Read the model definition and answer for the solid it produces. Units are mm, in the model's axes. A direction names the side the tool comes from. Coordinates: 2 decimals unless noted, no trailing zeros. Loops run counter-clockwise (first coordinate to the right, second up) from the corner with the lowest first, then second, coordinate; pieces in that order, holes last. Notation, with made-up numbers: (-23, 47.5) - (1, 47.5) arc R32 cw to (1, 86.5) - close; hole circle Ø7 at (66.5, -38). An arc over 180 degrees is marked (long way). Use CSV: the item, a comma, the result in double quotes.
```python
from build123d import *

# Parameters (mm, degrees)
BOSS_EXTRUDE1_DEPTH = 7.9
SKETCH4_W           = 6.315653724
SKETCH4_H           = 4.166384482
CUT_EXTRUDE2_DEPTH  = 1.6
SHELL1_T            = -0.5
SKETCH2_W           = 0.603812539
SKETCH2_H           = 7.583931724
CUT_EXTRUDE1_DEPTH  = 1.55
SKETCH5_W           = 0.832806424
SKETCH5_H           = 1.205065976
CUT_EXTRUDE3_DEPTH  = 0.25
SKETCH6_W           = 9.378889646
SKETCH6_H           = 1.1
CUT_EXTRUDE4_DEPTH  = 0.25


with BuildPart() as part:
    # Sketch1 → Boss-Extrude1 (new body)
    with BuildSketch(Plane(origin=(0, 0, 0), x_dir=(0, 0, -1), z_dir=(1, 0, 0))):
        Polygon((0, 0), (0, -3.3), (7.6, -3.3), (7.6, -1.216807759), (6, 0), (6, 2.2), (0, 2.2), align=None)
    extrude(amount=BOSS_EXTRUDE1_DEPTH)

    # Sketch4 → Cut-Extrude2 (cut)
    with BuildSketch(Plane(origin=(0, 0, -7.6), x_dir=(-1, 0, 0), z_dir=(0, 0, -1))):
        with Locations((-3.95, -1.216807759)):
            Rectangle(SKETCH4_W, SKETCH4_H)
    extrude(amount=-CUT_EXTRUDE2_DEPTH, mode=Mode.SUBTRACT)

    # Shell1
    shell1_openings = [part.faces().sort_by_distance(p)[0] for p in [
        (3.95, -0.55, 0),
    ]]
    offset(amount=SHELL1_T, openings=shell1_openings, kind=Kind.INTERSECTION)

    # Sketch2 → Cut-Extrude1 (cut)
    with BuildSketch(Plane(origin=(0, 2.2, 0), x_dir=(1, 0, 0), z_dir=(0, 1, 0))):
        with Locations((5.978601851, 6)):
            Rectangle(SKETCH2_W, SKETCH2_H)
        with Locations((1.92139815, 6)):
            Rectangle(SKETCH2_W, SKETCH2_H)
    extrude(amount=-CUT_EXTRUDE1_DEPTH, mode=Mode.SUBTRACT)

    # Sketch5 → Cut-Extrude3 (cut)
    with BuildSketch(Plane(origin=(0, 2.2, 0), x_dir=(1, 0, 0), z_dir=(0, 1, 0))):
        with Locations((1.428135285, 0)):
            Rectangle(SKETCH5_W, SKETCH5_H)
    extrude(amount=-CUT_EXTRUDE3_DEPTH, mode=Mode.SUBTRACT)

    # Sketch6 → Cut-Extrude4 (cut)
    with BuildSketch(Plane.ZY):
        with Locations((0, -0.55)):
            Rectangle(SKETCH6_W, SKETCH6_H)
    cut_extrude4 = extrude(amount=-CUT_EXTRUDE4_DEPTH, mode=Mode.SUBTRACT)

    # Mirror1: Cut-Extrude4 across plane
    add(cut_extrude4.mirror(Plane.ZY.offset(-3.95)), mode=Mode.SUBTRACT)


solid = part.part
```
Q1. Find the intervals of material crossed by probe 1 along X at (y, z) = (1.9, -4); probe 2 along X at (y, z) = (-0.2, -0.25); probe 3 along Y at (x, z) = (1.25, -3.75), in increasing order. Write a range as [from, to].
Reported:
probe 1,"x = [0, 1.62], [2.22, 5.68], [6.28, 7.9]"
probe 2,"x = [0.25, 0.5], [7.4, 7.65]"
probe 3,"y = [-3.3, -2.8], [1.7, 2.2]"
Q2. The part is cut by section D-D on z = -2. Determine the outline of the cut face in (x, y), and give its area (4 significant figures).
Reported:
outline,"(0, -3.3) - (7.9, -3.3) - (7.9, -1.1) - (7.65, -1.1) - (7.65, 0) - (7.9, 0) - (7.9, 2.2) - (0, 2.2) - (0, 0) - (0.25, 0) - (0.25, -1.1) - (0, -1.1) - close; hole (0.5, -2.8) - (7.4, -2.8) - (7.4, 1.7) - (0.5, 1.7) - close"
area,"11.85 mm²"
Q3. The part is cut by section C-C on x = 6. Determine the outline of the cut face in (y, z).
Reported:
outline,"(-3.3, -6) - (0.65, -6) - (0.65, -5.5) - (-2.8, -5.5) - (-2.8, 0) - (-3.3, 0) - close; (1.7, -2.21) - (2.2, -2.21) - (2.2, 0) - (1.7, 0) - close"
Q4. For a pull along Y with two mould halves and no side action, classify faces 5 (the face through (0.5, -1, -3)), 6 (the face through (4, 1.7, -3)), 7 (the face through (0.391, -0.617, -6.811)), 8 (the face through (1.619, 2, -4)) as +Y half, -Y half, draft (parallel to the pull), parting line (faces both ways), or undercut.
Reported:
face 5,"undercut"
face 6,"undercut"
face 7,"+Y half"
face 8,"draft"
Q5. Given P1, Ø0.6, axis at y = -0.5, z = -3, coming from the +X side, flat-ended and moving along its own axis, determine where the tip first touches the part or whether it passes through.
Reported:
P1,"stops at x = 7.65"
Q6. The part is cut by section B-B on y = 1.55. Determine the outline of the cut face in (x, z).
Reported:
outline,"(0, -6) - (1.62, -6) - (1.62, -5.5) - (0.5, -5.5) - (0.5, 0) - (0, 0) - close; (2.22, -6) - (5.68, -6) - (5.68, -5.5) - (2.22, -5.5) - close; (6.28, -6) - (7.9, -6) - (7.9, 0) - (7.4, 0) - (7.4, -5.5) - (6.28, -5.5) - close"
Q7. A tool of negligible diameter and unlimited length cuts with its end or side. For faces 1 (the face through (5.677, 2, -4)), 2 (the face through (4, -2.8, -3)), 3 (the face through (0.792, -2, -7)), 4 (the face through (7.65, -0.5, -2.4)), from which of +Z, -Z, +X, -X, +Y, -Y can it reach the whole face along a straight path? Write none if from no direction.
Reported:
face 1,"-Z, +Y"
face 2,"+Z"
face 3,"-Z, +Y, -Y"
face 4,"+Z, +X"
Q8. The part is cut by section A-A on z = -3.5. Determine the outline of the cut face in (x, y).
Reported:
outline,"(0, -3.3) - (7.9, -3.3) - (7.9, -1.1) - (7.65, -1.1) - (7.65, 0) - (7.9, 0) - (7.9, 2.2) - (6.28, 2.2) - (6.28, 1.7) - (7.4, 1.7) - (7.4, -2.8) - (0.5, -2.8) - (0.5, 1.7) - (1.62, 1.7) - (1.62, 2.2) - (0, 2.2) - (0, 0) - (0.25, 0) - (0.25, -1.1) - (0, -1.1) - close; (2.22, 1.7) - (5.68, 1.7) - (5.68, 2.2) - (2.22, 2.2) - close"
